Read the model definition and answer for the solid it produces. Units are mm, in the model's axes. A direction names the side the tool comes from. Coordinates: 2 decimals unless noted, no trailing zeros. Return JSON: item names as keys, results as strings.
```python
from build123d import *

# Parameters (mm, degrees)
AUFSATZ_LINEAR_AUSTRAGEN1_DEPTH      = 4
AUFSATZ_LINEAR_AUSTRAGEN1_DEPTH_BACK = 4
SKIZZE1_W                            = 287
SKIZZE1_H                            = 80
SCHNITT_LINEAR_AUSTRAGEN1_DEPTH      = 20
SCHNITT_LINEAR_AUSTRAGEN2_DEPTH      = 150.024326873
SCHNITT_LINEAR_AUSTRAGEN2_DEPTH_BACK = 150.024326873
VERRUNDUNG1_R                        = 4
VERRUNDUNG2_R                        = 1
FASE1_SIZE                           = 1


with BuildPart() as part:
    # Skizze1 → Aufsatz-Linear austragen1 (new, two sides: drawn at the far end of the back side and taken through both)
    with BuildSketch(Plane.XY.offset(-AUFSATZ_LINEAR_AUSTRAGEN1_DEPTH_BACK)):
        Rectangle(SKIZZE1_W, SKIZZE1_H)
    extrude(amount=AUFSATZ_LINEAR_AUSTRAGEN1_DEPTH + AUFSATZ_LINEAR_AUSTRAGEN1_DEPTH_BACK)

    # Skizze2 → Schnitt-Linear austragen1 (cut)
    with BuildSketch(Plane.ZY.offset(143.5)):
        Polygon((1.25, 35), (0, 36.25), (-1.25, 35), (0, 33.75), align=None)
        Polygon((-1.25, -35), (0, -33.75), (1.25, -35), (0, -36.25), align=None)
    schnitt_linear_austragen1 = extrude(amount=-SCHNITT_LINEAR_AUSTRAGEN1_DEPTH, mode=Mode.SUBTRACT)

    # Spiegeln1: Schnitt-Linear austragen1 across plane
    add(schnitt_linear_austragen1.mirror(Plane(origin=(0, 0, 0), x_dir=(0, 0, 1), z_dir=(1, 0, 0))), mode=Mode.SUBTRACT)

    # Skizze3 → Schnitt-Linear austragen2 (cut, two sides: drawn at the far end of the back side and taken through both)
    with BuildSketch(Plane.XY.offset(-SCHNITT_LINEAR_AUSTRAGEN2_DEPTH_BACK)):
        Polygon((-114.526468265, 34), (-2, 34), (-2, 2.633737069), align=None)
        Polygon((-137.5, 31), (-137.5, 0), (-137.5, -31), (-118.661031735, -31), (-7.448531735, 0), (-118.661031735, 31), align=None)
        Polygon((-2, -34), (-2, -2.633737069), (-114.526468265, -34), align=None)
        Polygon((118.661031735, -31), (137.5, -31), (137.5, 0), (137.5, 31), (118.661031735, 31), (7.448531735, 0), align=None)
        Polygon((114.526468265, -34), (2, -34), (2, -2.633737069), align=None)
        Polygon((2, 2.633737069), (114.526468265, 34), (2, 34), align=None)
    extrude(amount=SCHNITT_LINEAR_AUSTRAGEN2_DEPTH + SCHNITT_LINEAR_AUSTRAGEN2_DEPTH_BACK, mode=Mode.SUBTRACT)

    # Verrundung1
    verrundung1_edges = [part.edges().sort_by_distance(p)[0] for p in [
        (2, -2.633737069, 0),
        (2, -34, 0),
        (137.5, 31, 0),
        (137.5, -31, 0),
        (2, 2.633737069, 0),
        (2, 34, 0),
        (-2, 2.633737069, 0),
        (-2, 34, 0),
        (-2, -34, 0),
        (-2, -2.633737069, 0),
        (-137.5, -31, 0),
        (-137.5, 31, 0),
    ]]
    fillet(verrundung1_edges, radius=VERRUNDUNG1_R)

    # Verrundung2
    verrundung2_edges = [part.edges().sort_by_distance(p)[0] for p in [
        (-7.448531735, 0, 0),
        (114.526468265, -34, 0),
        (7.448531735, 0, 0),
        (114.526468265, 34, 0),
        (-114.526468265, 34, 0),
        (-114.526468265, -34, 0),
    ]]
    fillet(verrundung2_edges, radius=VERRUNDUNG2_R)

    # Fase1
    fase1_edges = [part.edges().sort_by_distance(p)[0] for p in [
        (0, -40, -4),
        (-64.782660021, -15.981638547, -4),
        (-64.782660021, -15.981638547, 4),
        (-126.080515867, 31, 4),
        (64.782660021, 15.981638547, -4),
        (126.080515867, -31, -4),
        (126.080515867, -31, 4),
        (64.782660021, 15.981638547, 4),
        (0, 40, 4),
        (0, -40, 4),
        (137.5, 0, -4),
        (137.5, 0, 4),
        (126.080515867, 31, -4),
        (126.080515867, 31, 4),
        (56.607351199, -34, -4),
        (56.607351199, -34, 4),
        (2, -18.950605603, -4),
        (2, -18.950605603, 4),
        (57.278624435, 18.04241287, -4),
        (57.278624435, 18.04241287, 4),
        (2, 18.950605603, -4),
        (2, 18.950605603, 4),
        (-2, 18.950605603, -4),
        (-2, 18.950605603, 4),
        (-57.278624435, -18.04241287, -4),
        (-57.278624435, -18.04241287, 4),
        (-2, -18.950605603, -4),
        (-2, -18.950605603, 4),
        (-56.607351199, 34, -4),
        (-56.607351199, 34, 4),
        (-126.080515867, -31, -4),
        (-126.080515867, -31, 4),
        (-137.5, 0, -4),
        (-137.5, 0, 4),
        (136.328427125, -29.828427125, 4),
        (136.328427125, -29.828427125, -4),
        (136.328427125, 29.828427125, 4),
        (136.328427125, 29.828427125, -4),
        (3.171572875, -32.828427125, 4),
        (3.171572875, -32.828427125, -4),
        (3.58092463, -4.71560697, 4),
        (3.58092463, -4.71560697, -4),
        (3.58092463, 4.71560697, 4),
        (3.58092463, 4.71560697, -4),
        (3.171572875, 32.828427125, 4),
        (3.171572875, 32.828427125, -4),
        (-3.58092463, 4.71560697, 4),
        (-3.58092463, 4.71560697, -4),
        (-3.58092463, -4.71560697, 4),
        (-3.58092463, -4.71560697, -4),
        (-3.171572875, -32.828427125, 4),
        (-3.171572875, -32.828427125, -4),
        (-3.171572875, 32.828427125, 4),
        (-3.171572875, 32.828427125, -4),
        (-136.328427125, -29.828427125, 4),
        (-136.328427125, -29.828427125, -4),
        (-136.328427125, 29.828427125, 4),
        (-136.328427125, 29.828427125, -4),
        (57.278624435, -18.04241287, 4),
        (57.278624435, -18.04241287, -4),
        (56.607351199, 34, 4),
        (56.607351199, 34, -4),
        (64.782660021, -15.981638547, -4),
        (64.782660021, -15.981638547, 4),
        (-64.782660021, 15.981638547, -4),
        (-64.782660021, 15.981638547, 4),
        (-56.607351199, -34, 4),
        (-56.607351199, -34, -4),
        (-57.278624435, 18.04241287, 4),
        (-57.278624435, 18.04241287, -4),
        (108.205479137, -33.13550444, 4),
        (108.205479137, -33.13550444, -4),
        (108.205479137, 33.13550444, 4),
        (108.205479137, 33.13550444, -4),
        (10.172797602, 0, 4),
        (10.172797602, 0, -4),
        (-10.172797602, 0, 4),
        (-10.172797602, 0, -4),
        (-108.205479137, -33.13550444, 4),
        (-108.205479137, -33.13550444, -4),
        (-108.205479137, 33.13550444, 4),
        (-108.205479137, 33.13550444, -4),
        (0, 40, -4),
        (-126.080515867, 31, -4),
    ]]
    chamfer(fase1_edges, length=FASE1_SIZE)


solid = part.part
```
(1) A flat-ended cylindrical pin translates along its axis: P1, Ø2, axis at y = -35, z = 0.5, coming from the -X side. Find the tip coordinate at first contact, or state that the pin passes through.
Answer:
{"P1": "x = -143.5"}
(2) Straight lines are drawn through the part: line 1 (Y direction, x = 7, z = 0.75); line 2 (Y direction, x = 39, z = -1); line 3 (Y direction, x = 83, z = 2). For each, find the intervals that lie inside material, in ascending order. Write a range as from..to.
Answer:
{"line 1": "-40..-34, -4.03..4.03, 34..40", "line 2": "-40..-34, -12.95..-8.79, 8.79..12.95, 34..40", "line 3": "-40..-34, -25.21..-21.06, 21.06..25.21, 34..40"}
(3) Determine the mould class of faces 1 (the face through (-22, -6, -4)), 2 (the face through (-57, -34, 0)) for opening direction X: +X half, -X half, draft (parallel to the pull), parting line (faces both ways), or undercut.
Answer:
{"face 1": "draft", "face 2": "undercut"}
(4) Which of the six approach directions +Z, -Z, +X, -X, +Y, -Y give full straight-line access (tool end or side, diameter ignored) to faces 3 (the face through (-2, 19, 0)), 4 (the face through (-58.114, -17.763, -3.493)), 5 (the face through (2.937, 32.996, 3.285))?
Answer:
{"face 3": "+Z, -Z", "face 4": "-Z", "face 5": "+Z"}
(5) A cutting plane is placed at A-A (x = -16.5). State how many separate pieces and enclosed holes the cut face has, and give its area (3 significant figures).
Answer:
{"separate pieces": "4", "enclosed holes": "0", "area": "154 mm²"}
